Geometry: see drawing. Coordinates: mm, zero at the bounding-box minimum. Give positions to 0.01 mm unless a question says otherwise; leave off trailing zeros. Order: outer loops, then holes, each group sorted by start corner. A loop starts at its lowest first (then second) coordinate and runs counter-clockwise, first axis right, second up. Notation, with made-up numbers: (15.25, 34) - (44.25, 34) arc R18 ccw to (44.25, 53) - close; hole circle Ø1 at (-26.75, -32.5). An arc over 180 degrees is marked (long way). One line per item, written item: value.
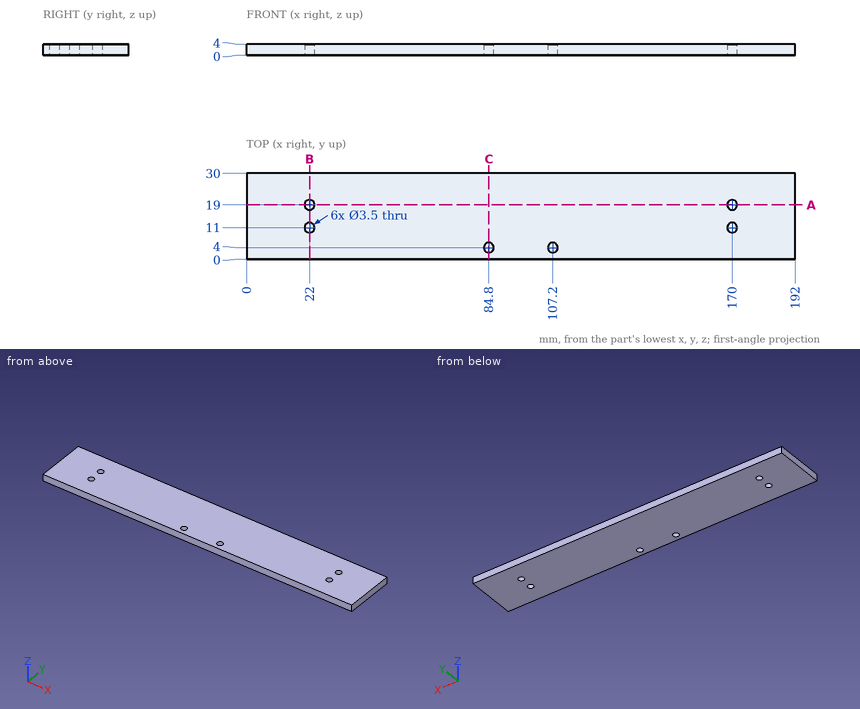
1) Material intervals for line 1 along X through (y, z) = (19.25, 3.75); line 2 along Y through (x, z) = (107.2, 2.25); line 3 along Y through (x, z) = (170, 1.1), sorted ascending.
Answers below:
line 1: 0 to 20.27, 23.73 to 168.27, 171.73 to 192
line 2: 0 to 2.25, 5.75 to 30
line 3: 0 to 9.25, 12.75 to 17.25, 20.75 to 30
2) Section A-A, the plane y = 19. Return loops of the section in (x, z), then the cut area to 3 significant figures.
Answers below:
outline: (0, 0) - (20.25, 0) - (20.25, 4) - (0, 4) - close; (23.75, 0) - (168.25, 0) - (168.25, 4) - (23.75, 4) - close; (171.75, 0) - (192, 0) - (192, 4) - (171.75, 4) - close
area: 740 mm^2
3) First-contact query: pin 1 (3 mm diameter, centred on x = 22, y = 19, fed in from +Z). Flat tip, straight axial feed; report the tip coordinate or a pass-through.
Answers below:
pin 1: through
4) Section B-B, the plane x = 22. Return loops of the section in (y, z), then the cut area to 3 significant figures.
Answers below:
outline: (0, 0) - (9.25, 0) - (9.25, 4) - (0, 4) - close; (12.75, 0) - (17.25, 0) - (17.25, 4) - (12.75, 4) - close; (20.75, 0) - (30, 0) - (30, 4) - (20.75, 4) - close
area: 92.0 mm^2
5) Section C-C, the plane x = 84.8. Return loops of the section in (y, z), then the cut area to 3 significant figures.
Answers below:
outline: (0, 0) - (2.25, 0) - (2.25, 4) - (0, 4) - close; (5.75, 0) - (30, 0) - (30, 4) - (5.75, 4) - close
area: 106 mm^2
